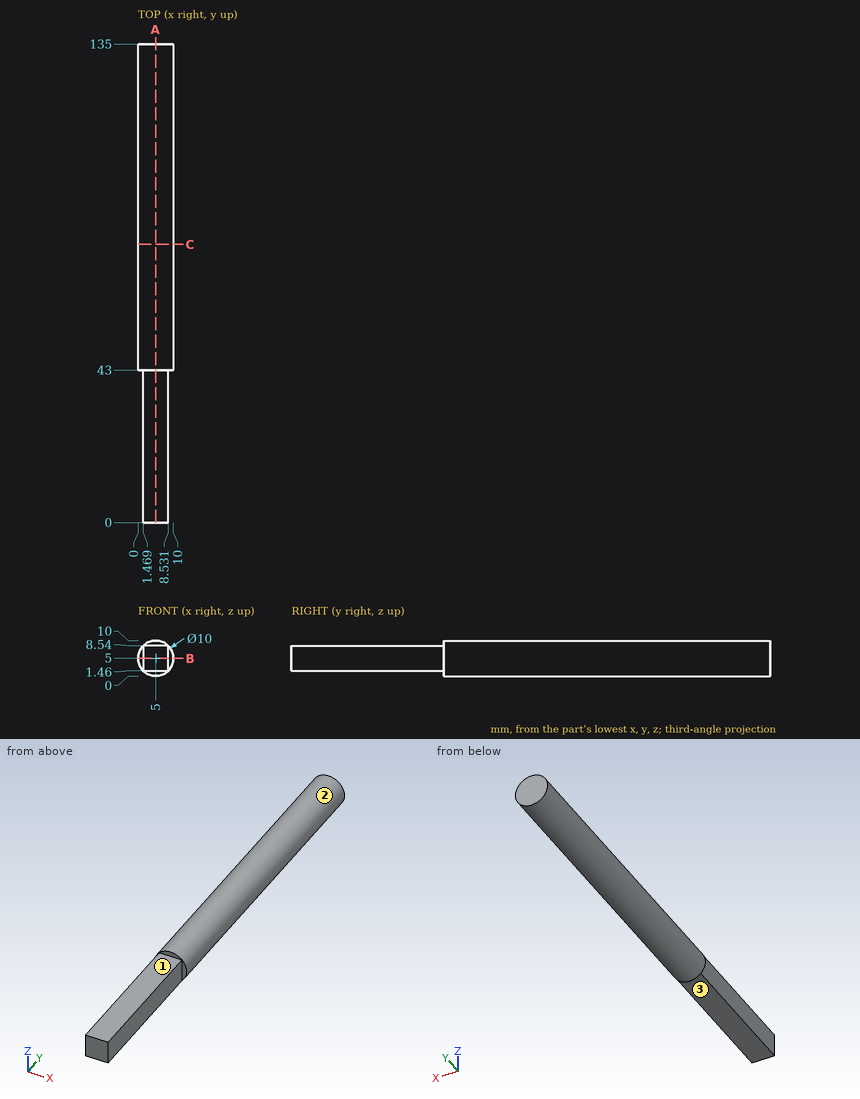
Study the drawing (mm; zero at the part's minimum x, y, z) and answer. A direction names the side the tool comes from. Coordinates: 2 decimals unless noted, no trailing zeros. Write each loop counter-clockwise with the first axis right and the second up, starting at its lowest first coordinate (ties: lowest second). Pieces come first, ordered by that corner, then holes.
Q1. Find the intervals of material crossed by line 1 (Y direction, x = 9.75, z = 5); line 2 (Z direction, x = 5.5, y = 24.5); line 3 (X direction, y = 63.5, z = 5.25), in increasing order.
Q2. Which of the six approach directions +Z, -Z, +X, -X, +Y, -Y give full straight-line access (tool end or side, diameter ignored) to the marked faces 1, 2 and 3?
Q3. A cutting plane is placed at A-A, the plane x = 5. Give the vertices of the cut face in (y, z), then the cut area to 3 significant figures.
Q4. A cutting plane is placed at B-B, the plane z = 5. Give the vertices of the cut face in (x, y), then the cut area to 3 significant figures.
Q5. A cutting plane is placed at C-C, the plane y = 78.5. Give the vertices of the cut face in (x, z), then the cut area to 3 significant figures.
Q6. Each of these flat-tipped pins is pushed along its axis until it touches: pin 1 Ø3.5 at (y, z) = (30, 4) entering from +X; pin 2 Ø1.6 at (x, z) = (4.5, 0.5) entering from -Y; pin 3 Ø3.5 at (y, z) = (20, 6.5) entering from -X. Where does it stop, or does it pass through?
Findings below:
1. line 1: y = 43 to 135
1. line 2: z = 1.46 to 8.54
1. line 3: x = 0.01 to 9.99
2. face 1: +Z, +X, -X, -Y
2. face 2: +Y, -Y
2. face 3: -Z, +X, -X, -Y
3. outline: (0, 1.46) - (43, 1.46) - (43, 0) - (135, 0) - (135, 10) - (43, 10) - (43, 8.54) - (0, 8.54) - close
3. area: 1,220 mm2
4. outline: (0, 43) - (1.47, 43) - (1.47, 0) - (8.53, 0) - (8.53, 43) - (10, 43) - (10, 135) - (0, 135) - close
4. area: 1,220 mm2
5. outline: circle Ø10 at (5, 5)
5. area: 78.5 mm2
6. pin 1: stops at x = 8.53
6. pin 2: stops at y = 43
6. pin 3: stops at x = 1.47
